from build123d import *

# Parameters (mm, degrees)
SKETCH1_R                 = 15
BOSS_EXTRUDE1_DEPTH       = 5
SKETCH2_R                 = 5
BOSS_EXTRUDE2_DEPTH       = 12.7
SKETCH3_R                 = 2
CUT_EXTRUDE1_DEPTH        = 9.5
SKETCH5_R                 = 1.25
CUT_EXTRUDE2_DEPTH        = 5
CIRPATTERN1_COUNT         = 4
M3X0_5_TAPPED_HOLE1_D     = 2.5
M3X0_5_TAPPED_HOLE2_D     = 2.5
M3X0_5_TAPPED_HOLE2_DEPTH = 4.999
M3X0_5_TAPPED_HOLE2_TIP   = 0.751075774
SKETCH12_R                = 4
BOSS_EXTRUDE3_DEPTH       = 23


with BuildPart() as part:
    # Sketch1 → Boss-Extrude1 (new body)
    with BuildSketch(Plane(origin=(0, 0, 0), x_dir=(1, 0, 0), z_dir=(0, 1, 0))):
        Circle(SKETCH1_R)
    extrude(amount=BOSS_EXTRUDE1_DEPTH)

    # Sketch2 → Boss-Extrude2 (add)
    with BuildSketch(Plane.XZ):
        Circle(SKETCH2_R)
    extrude(amount=BOSS_EXTRUDE2_DEPTH)

    # Sketch3 → Cut-Extrude1 (cut)
    with BuildSketch(Plane.XZ.offset(12.7)):
        Circle(SKETCH3_R)
    extrude(amount=-CUT_EXTRUDE1_DEPTH, mode=Mode.SUBTRACT)

    # Sketch5 → Cut-Extrude2 (cut)
    with BuildSketch(Plane(origin=(0, 5, 0), x_dir=(1, 0, 0), z_dir=(0, 1, 0))):
        with Locations((0, -10)):
            Circle(SKETCH5_R)
    cut_extrude2 = extrude(amount=-CUT_EXTRUDE2_DEPTH, mode=Mode.SUBTRACT)

    # CirPattern1: Cut-Extrude2 ×4 about axis
    cirpattern1_axis = Axis((0, 0, 0), (0, 1, 0))
    for i in range(1, CIRPATTERN1_COUNT):
        add(cut_extrude2.rotate(cirpattern1_axis, i * 360 / CIRPATTERN1_COUNT), mode=Mode.SUBTRACT)

    # M3x0.5 Tapped Hole1 (through all)
    with Locations(Plane(origin=(0, 5, 0), x_dir=(1, 0, 0), z_dir=(0, 1, 0))):
        with Locations((-10, 0), (0, -10), (10, 0), (0, 10)):
            Hole(M3X0_5_TAPPED_HOLE1_D / 2)

    # M3x0.5 Tapped Hole2
    with Locations(Plane.XY.offset(5)):
        with Locations((0, -8.7)):
            Hole(M3X0_5_TAPPED_HOLE2_D / 2, depth=M3X0_5_TAPPED_HOLE2_DEPTH)
            with Locations((0, 0, -(M3X0_5_TAPPED_HOLE2_DEPTH + M3X0_5_TAPPED_HOLE2_TIP / 2))):  # 118° drill point
                Cone(0, M3X0_5_TAPPED_HOLE2_D / 2, M3X0_5_TAPPED_HOLE2_TIP, mode=Mode.SUBTRACT)

    # Sketch12 → Boss-Extrude3 (add)
    with BuildSketch(Plane(origin=(0, 5, 0), x_dir=(1, 0, 0), z_dir=(0, 1, 0))):
        Circle(SKETCH12_R)
    extrude(amount=BOSS_EXTRUDE3_DEPTH)


solid = part.part
The listing builds one solid part. Answer for the finished solid, in the listing's coordinates (mm). A direction names the side the tool comes from. Give positions to 0.01 mm unless a question says otherwise; leave off trailing zeros. Write each loop counter-clockwise with the first axis right and the second up, starting at its lowest first coordinate (ties: lowest second). Pieces come first, ordered by that corner, then holes. Notation, with made-up numbers: (36, 79.25) - (60, 79.25) arc R21 cw to (60, 100.25) - close; hole circle Ø7 at (34, 12.25). An arc over 180 degrees is marked (long way). Use a Markdown table: item, result.
1. Section A-A on z = 0 is taken. Write down the section's boundary in (x, y).
Values follow:
| item | result |
|---|---|
| outline | (-15, 0) - (-11.25, 0) - (-11.25, 5) - (-15, 5) - close; (-8.75, 0) - (-5, 0) - (-5, -12.7) - (-2, -12.7) - (-2, -3.2) - (2, -3.2) - (2, -12.7) - (5, -12.7) - (5, 0) - (8.75, 0) - (8.75, 5) - (4, 5) - (4, 28) - (-4, 28) - (-4, 5) - (-8.75, 5) - close; (11.25, 0) - (15, 0) - (15, 5) - (11.25, 5) - close |
2. Find the intervals of material crossed by probe 1 along Z at (x, y) = (0, 2.65); probe 2 along Y at (x, z) = (-4, -0.5); probe 3 along Z at (x, y) = (0, -5.5), in increasing order. Write a range as from..to.
Values follow:
| item | result |
|---|---|
| probe 1 | z = -15..-11.25, -8.75..8.75, 11.25..15 |
| probe 2 | y = -12.7..5 |
| probe 3 | z = -5..-2, 2..5 |
3. For a pull along Y with two mould halves and no side action, classify faces 1 (the cylindrical face through (-1.19, -8.32, 3.26)), 2 (the flat face through (3, 5, 3)), 3 (the cylindrical face through (-0.867, 16.339, 3.905)) as released by +Y, released by -Y, zero draft, split by the parting line, or undercut.
Values follow:
| item | result |
|---|---|
| face 1 | undercut |
| face 2 | released by +Y |
| face 3 | zero draft |
4. Section B-B on x = 0 is taken. Write down the section's boundary in (y, z), plus the area to 4 significant figures.
Values follow:
| item | result |
|---|---|
| outline | (-12.7, -5) - (0, -5) - (0, -8.75) - (5, -8.75) - (5, -4) - (28, -4) - (28, 4) - (5, 4) - (5, 8.75) - (0, 8.75) - (0, 5) - (-7.45, 5) - (-7.45, 2) - (-3.2, 2) - (-3.2, -2) - (-12.7, -2) - close; (-12.7, 2) - (-9.95, 2) - (-9.95, 5) - (-12.7, 5) - close; (0, -15) - (5, -15) - (5, -11.25) - (0, -11.25) - close; (0, 11.25) - (5, 11.25) - (5, 15) - (0, 15) - close |
| area | 390.5 mm² |
5. Section D-D on x = 10 is taken. Write down the section's boundary in (y, z).
Values follow:
| item | result |
|---|---|
| outline | (0, -11.18) - (5, -11.18) - (5, -1.25) - (0, -1.25) - close; (0, 1.25) - (5, 1.25) - (5, 11.18) - (0, 11.18) - close |
6. Section C-C on z = 10 is taken. Write down the section's boundary in (x, y), plus the area to 3 significant figures.
Values follow:
| item | result |
|---|---|
| outline | (-11.18, 0) - (-1.25, 0) - (-1.25, 5) - (-11.18, 5) - close; (1.25, 0) - (11.18, 0) - (11.18, 5) - (1.25, 5) - close |
| area | 99.3 mm² |
7. A tool of negligible diameter and unlimited length cuts with its end or side. For faces 4 (the cylindrical face through (8.946, 2.535, -0.672)), 5 (the cylindrical face through (0, -8, -2)), from which of +Z, -Z, +X, -X, +Y, -Y can it reach the whole face along a straight path? Write none if from no direction.
Values follow:
| item | result |
|---|---|
| face 4 | +Y, -Y |
| face 5 | -Y |
8. Each of these flat-tipped pins is pushed along its axis until it touches: P1, Ø4, axis at x = 0, z = 10, coming from the -Y side; P2, Ø6, axis at y = -5.5, z = -0.5, coming from the -X side; P3, Ø9, axis at x = 7, z = 5.5, coming from the +Y side; P4, Ø4, axis at y = -3, z = 10.5, coming from the +X side. Where does it stop, or does it pass through?
Values follow:
| item | result |
|---|---|
| P1 | stops at y = 0 |
| P2 | stops at x = -5 |
| P3 | stops at y = 5 |
| P4 | passes through |
